from build123d import *

# Parameters (mm, degrees)
F2_R = 0.5


with BuildPart() as f1:
    # F0 (on Right) → F1 (revolve)
    with BuildSketch(Plane.YZ):
        Polygon((-8.75, 7.5), (-12, 7.5), (-12, 4), (12, 4), (12, 7.5), (9.85, 7.5), (9.85, 7.15), (8.75, 7.15), (8.75, 7.5), (-7.65, 7.5), (-7.65, 7.15), (-8.75, 7.15), align=None)
    revolve(axis=Axis((0, 2.064935, 0), (0, 1, 0)))

    # F2
    f2_edges = [f1.edges().sort_by_distance(p)[0] for p in [
        (0, 12, -7.5),
        (0, -12, -7.5),
    ]]
    fillet(f2_edges, radius=F2_R)


solid = f1.part
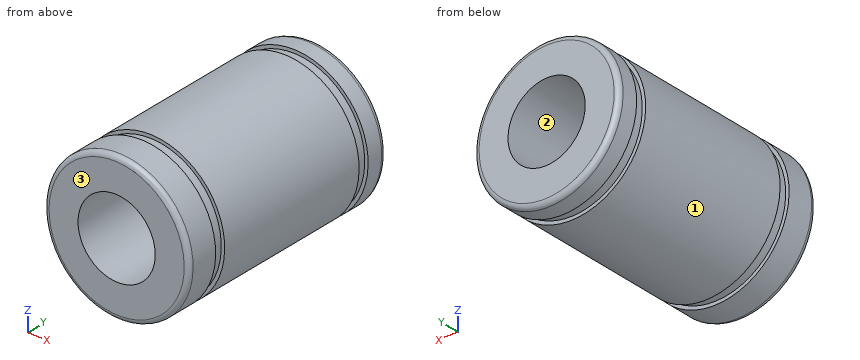
Read the model definition and answer for the solid it produces. Units are mm, in the model's axes. Face numbers are marked on the shaded views. Coordinates: 2 decimals unless noted, no trailing zeros. Loops run counter-clockwise (first coordinate to the right, second up) from the corner with the lowest first, then second, coordinate; pieces in that order, holes last. Notation, with made-up numbers: (35, 66.25) -> (92, 66.25) arc R35 ccw to (92, 99.25) -> close; hole circle Ø11 at (-10, -33.75). An arc over 180 degrees is marked (long way). Write item = value, one per line. Start each with the question number.
1) The part is cut by section B-B, the plane x = 0. Determine the outline of the cut face in (y, z).
2) Find the intervals of material crossed by L1, parallel to X at y = -5.25, z = 0; L2, parallel to Z at x = 3, y = -3; L3, parallel to Z at x = -1.5, y = 10.75, in increasing order. Write a range as from..to.
3) The part is cut by section C-C, the plane y = -9.5. Determine the outline of the cut face in (x, z), plus the area to 3 significant figures.
4) Given P1, Ø5, axis at x = 0, z = 0, coming from the -Y side; P2, Ø5, axis at x = 5, y = 5, coming from the +Z side; P3, Ø3, axis at x = -3.5, y = -8.5, coming from the +Z side, each flat-ended and moving along its own axis, determine where each tip first touches the part or whether it passes through.
5) The mould has two halves that part along Z. Classify the marked faces 1, 2 and 3: pulls with the +Z half, pulls with the -Z half, needs draft (parallel to the pull), parting line crosses it, or undercut.
6) The part is cut by section A-A, the plane z = 0. Determine the outline of the cut face in (x, y), plus the area to 3 significant figures.
Result:
q1.outline = (-12, -7) arc R0.5 ccw to (-11.5, -7.5) -> (-8.75, -7.5) -> (-8.75, -7.15) -> (-7.65, -7.15) -> (-7.65, -7.5) -> (8.75, -7.5) -> (8.75, -7.15) -> (9.85, -7.15) -> (9.85, -7.5) -> (11.5, -7.5) arc R0.5 ccw to (12, -7) -> (12, -4) -> (-12, -4) -> close; (-12, 4) -> (12, 4) -> (12, 7) arc R0.5 ccw to (11.5, 7.5) -> (9.85, 7.5) -> (9.85, 7.15) -> (8.75, 7.15) -> (8.75, 7.5) -> (-7.65, 7.5) -> (-7.65, 7.15) -> (-8.75, 7.15) -> (-8.75, 7.5) -> (-11.5, 7.5) arc R0.5 ccw to (-12, 7) -> close
q2.L1 = -7.5..-4, 4..7.5
q2.L2 = -6.87..-2.65, 2.65..6.87
q2.L3 = -7.35..-3.71, 3.71..7.35
q3.outline = circle Ø15 at (0, 0); hole circle Ø8 at (0, 0)
q3.area = 126 mm²
q4.P1 = through
q4.P2 = 7.07
q4.P3 = 7.22
q5.face_1 = parting line crosses it
q5.face_2 = undercut
q5.face_3 = needs draft
q6.outline = (-7.5, -11.5) arc R0.5 ccw to (-7, -12) -> (-4, -12) -> (-4, 12) -> (-7, 12) arc R0.5 ccw to (-7.5, 11.5) -> (-7.5, 9.85) -> (-7.15, 9.85) -> (-7.15, 8.75) -> (-7.5, 8.75) -> (-7.5, -7.65) -> (-7.15, -7.65) -> (-7.15, -8.75) -> (-7.5, -8.75) -> close; (4, -12) -> (7, -12) arc R0.5 ccw to (7.5, -11.5) -> (7.5, -8.75) -> (7.15, -8.75) -> (7.15, -7.65) -> (7.5, -7.65) -> (7.5, 8.75) -> (7.15, 8.75) -> (7.15, 9.85) -> (7.5, 9.85) -> (7.5, 11.5) arc R0.5 ccw to (7, 12) -> (4, 12) -> close
q6.area = 166 mm²
